```python
from build123d import *

# Parameters (mm, degrees)
SKETCH_1_R          = 4
EXTRUDE_1_DEPTH     = 11.5
SKETCH_3_W          = 25
SKETCH_3_H          = 25
EXTRUDE_2_DEPTH     = 5
SKETCH_4_R          = 1.5
CUT_EXTRUDE_2_DEPTH = 5


with BuildPart() as part:
    # 草图1 → 凸台-拉伸1 (new body)
    with BuildSketch(Plane(origin=(0, 0, 0), x_dir=(1, 0, 0), z_dir=(0, 1, 0))):
        with Locations(Location((0, 0, 0), (0, 0, 270))):
            Circle(SKETCH_1_R)
    extrude(amount=EXTRUDE_1_DEPTH)

    # 草图3 → 凸台-拉伸2 (add)
    with BuildSketch(Plane.XZ):
        Rectangle(SKETCH_3_W, SKETCH_3_H)
    extrude(amount=EXTRUDE_2_DEPTH)

    # 草图4 → 切除-拉伸2 (cut)
    with BuildSketch(Plane(origin=(0, 0, 0), x_dir=(1, 0, 0), z_dir=(0, 1, 0))):
        with Locations(Location((9.5, 5, 0), (0, 0, 270))):
            Circle(SKETCH_4_R)
        with Locations(Location((9.5, -5, 0), (0, 0, 270))):
            Circle(SKETCH_4_R)
        with Locations(Location((-9.5, -5, 0), (0, 0, 270))):
            Circle(SKETCH_4_R)
        with Locations(Location((-9.5, 5, 0), (0, 0, 270))):
            Circle(SKETCH_4_R)
    extrude(amount=-CUT_EXTRUDE_2_DEPTH, mode=Mode.SUBTRACT)


solid = part.part
```
Source: CAD feature listing. Evaluate the final solid. Frame: model axes, mm. A direction names the side the tool comes from. Round coordinates to 2 decimals unless told otherwise and drop trailing zeros. Loops run counter-clockwise (first coordinate to the right, second up) from the corner with the lowest first, then second, coordinate; pieces in that order, holes last.
(1) Material intervals for probe 1 along X at (y, z) = (-3.25, -5); probe 2 along Y at (x, z) = (5.25, 7); probe 3 along X at (y, z) = (2, 0.75), sorted ascending.
From the geometry:
probe 1: x = -12.5 to -11, -8 to 8, 11 to 12.5
probe 2: y = -5 to 0
probe 3: x = -3.93 to 3.93
(2) Section query B-B (y = -1.75). Output: boundary loops of the cut face in (x, z), and give its area (3 significant figures).
From the geometry:
outline: (-12.5, -12.5) - (12.5, -12.5) - (12.5, 12.5) - (-12.5, 12.5) - close; hole circle Ø3 at (-9.5, -5); hole circle Ø3 at (-9.5, 5); hole circle Ø3 at (9.5, -5); hole circle Ø3 at (9.5, 5)
area: 597 mm2
(3) Section query A-A (x = -9.5). Output: boundary loops of the cut face in (y, z), and give its area (3 significant figures).
From the geometry:
outline: (-5, -12.5) - (0, -12.5) - (0, -6.5) - (-5, -6.5) - close; (-5, -3.5) - (0, -3.5) - (0, 3.5) - (-5, 3.5) - close; (-5, 6.5) - (0, 6.5) - (0, 12.5) - (-5, 12.5) - close
area: 95.0 mm2
(4) Contact query for flat-ended pins moving along their axis: pin 1 Ø1.8 at (x, z) = (-9.5, 5) entering from -Y; pin 2 Ø6 at (y, z) = (9.5, -2) entering from -X. Output: stop coordinate, or through.
From the geometry:
pin 1: passes through
pin 2: stops at x = -4
(5) Section query C-C (z = 0). Output: boundary loops of the cut face in (x, y).
From the geometry:
outline: (-12.5, -5) - (12.5, -5) - (12.5, 0) - (4, 0) - (4, 11.5) - (-4, 11.5) - (-4, 0) - (-12.5, 0) - close
(6) Access query for faces 1 (the flat face through (-3, 0, 3)), 2 (the flat face through (0, -2, -12.5)). Directions: +Z, -Z, +X, -X, +Y, -Y. A direction counts if a zero-diameter tool reaches every point of the face in a straight line with its end or side. Return the directions, or none.
From the geometry:
face 1: +Y
face 2: -Z, +X, -X, +Y, -Y
(7) Section query D-D (x = 0). Output: boundary loops of the cut face in (y, z), and give its area (3 significant figures).
From the geometry:
outline: (-5, -12.5) - (0, -12.5) - (0, -4) - (11.5, -4) - (11.5, 4) - (0, 4) - (0, 12.5) - (-5, 12.5) - close
area: 217 mm2
(8) Pull-direction query (Z, two-part tool) for faces 3 (the flat face through (-12.5, -2, 0)), 4 (the flat face through (0, -2, 12.5)), 5 (the cylindrical face through (-3.905, 5.67, -0.867)), 6 (the cylindrical face through (-10.83, -2.46, 5.69)); classes: +Z half, -Z half, draft (parallel to the pull), parting line (faces both ways), or undercut.
From the geometry:
face 3: draft
face 4: +Z half
face 5: parting line
face 6: undercut
